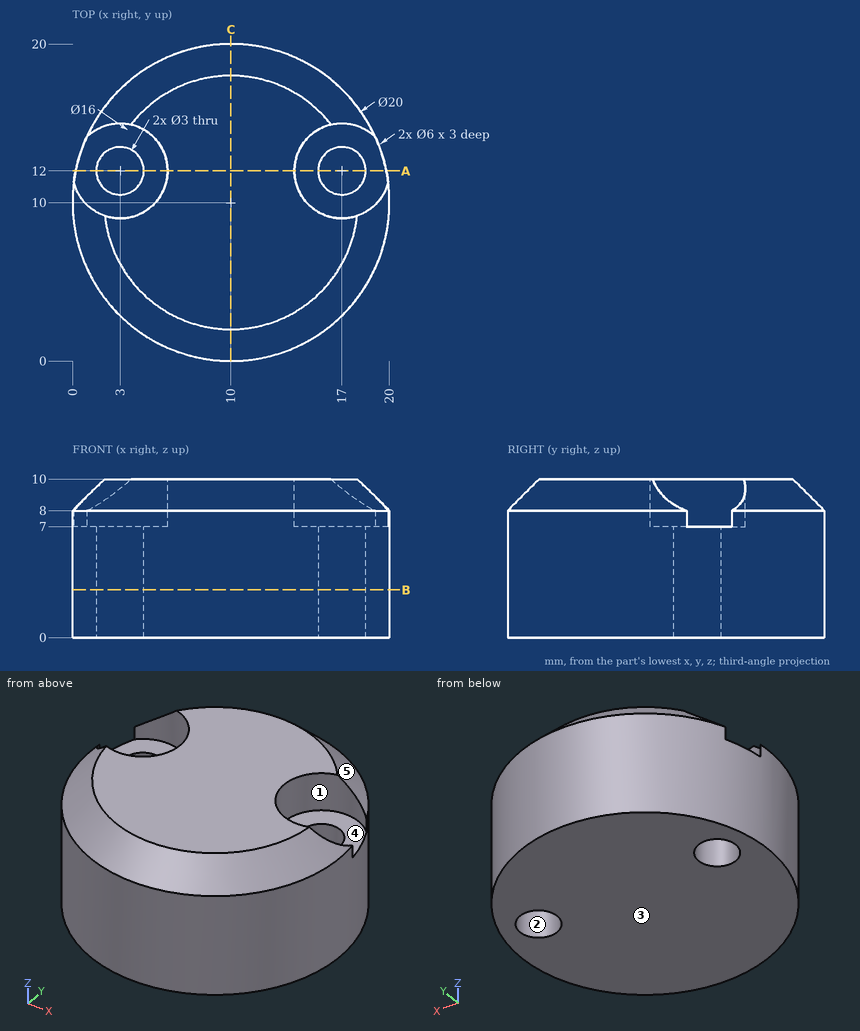
Geometry: see drawing. Coordinates: mm, zero at the bounding-box minimum. A direction names the side the tool comes from. Coordinates: 2 decimals unless noted, no trailing zeros. Order: outer loops, then holes, each group sorted by start corner. A loop starts at its lowest first (then second) coordinate and runs counter-clockwise, first axis right, second up. Notation, with made-up numbers: M 27,42.5 L 72,42.5 A3 cw 72,46.5 Z; hole C -22.75,45 d10. An arc over 180 degrees is marked long. Write item = value, one per line. Start each with the question number.
(1) Section B-B on z = 3. Output: boundary loops of the cut face in (x, y), and give its area (3 significant figures).
(2) Reachability of the marked faces 1 and 2 from +Z, -Z, +X, -X, +Y, -Y: full face, straight path, thin tool, end or side. Return the list, or none.
(3) First-contact query: P1, Ø5.5, axis at x = 3, y = 12, coming from the +Z side; P2, Ø3, axis at x = 12, z = 9, coming from the -Y side; P3, Ø1.8, axis at x = 17, y = 12, coming from the -Z side; P4, Ø2, axis at y = 2.5, z = 1.5, coming from the -X side. Flat tips, straight axial feed; report the tip coordinate or a pass-through.
(4) Line query: line 1 along Y through (x, z) = (17, 3); line 2 along X through (y, z) = (12.75, 5); line 3 along Y through (x, z) = (3, 7.8). Output: solid intervals per line, ascending. Write a range as [from, to].
(5) Pull-direction query (X, two-part tool) for the marked faces 3, 4 and 5; classes: released by +X, released by -X, zero draft, split by the parting line, or undercut.
(6) Section C-C on x = 10. Output: boundary loops of the cut face in (y, z).
(7) Section A-A on y = 12. Output: boundary loops of the cut face in (x, z), and give its area (3 significant figures).
Result set:
q1.outline = C 10,10 d20; hole C 3,12 d3; hole C 17,12 d3
q1.area = 300 mm²
q2.face_1 = +Z
q2.face_2 = +Z, -Z
q3.P1 = 7
q3.P2 = 0.04
q3.P3 = through
q3.P4 = 2.4
q4.line_1 = [2.86, 10.5], [13.5, 17.14]
q4.line_2 = [0.39, 1.7], [4.3, 15.7], [18.3, 19.61]
q4.line_3 = [2.86, 9], [15, 17.14]
q5.face_3 = zero draft
q5.face_4 = undercut
q5.face_5 = split by the parting line
q6.outline = M 0,0 L 20,0 L 20,8 L 18,10 L 2,10 L 0,8 Z
q7.outline = M 0.2,0 L 1.5,0 L 1.5,7 L 0.2,7 Z; M 4.5,0 L 15.5,0 L 15.5,7 L 14,7 L 14,10 L 6,10 L 6,7 L 4.5,7 Z; M 18.5,0 L 19.8,0 L 19.8,7 L 18.5,7 Z
q7.area = 119 mm²
